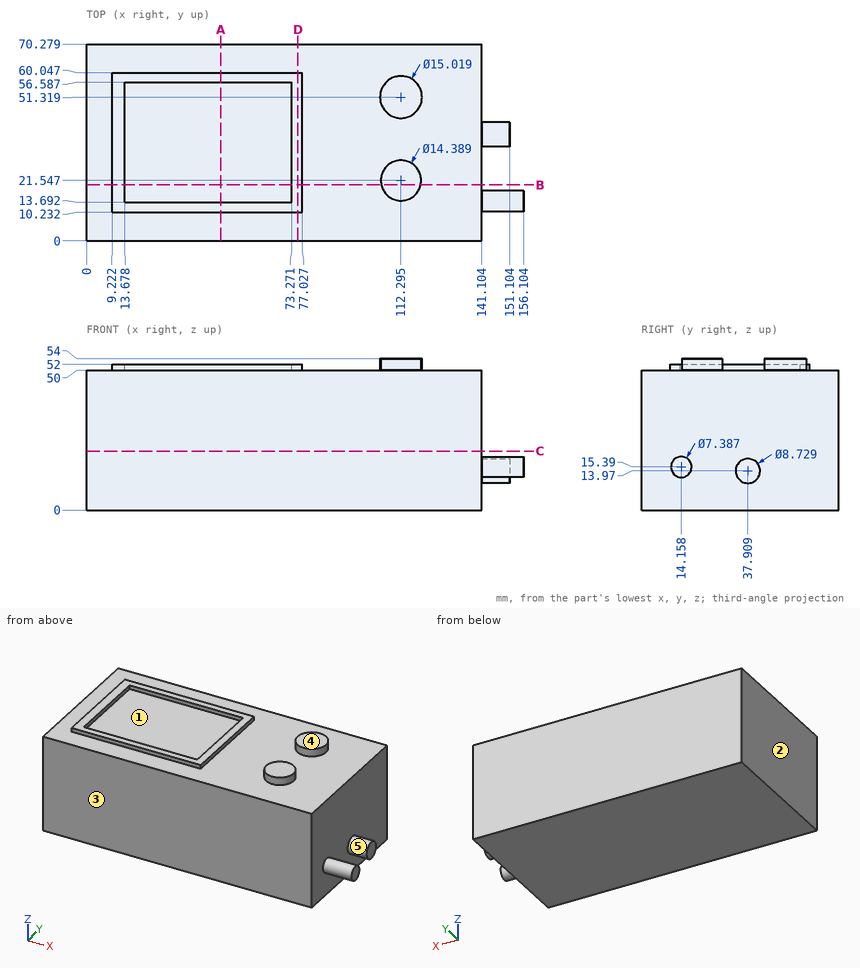
The drawing under review shows one solid part. Ordinate dimensions are in mm from its lowest x, y, z. A direction names the side the tool comes from. Give positions to 0.01 mm unless a question says otherwise; leave off trailing zeros. Write each loop counter-clockwise with the first axis right and the second up, starting at its lowest first coordinate (ties: lowest second). Pieces come first, ordered by that corner, then holes. Notation, with made-up numbers: (-11.5, -2) -> (12.5, -2) arc R37 cw to (12.5, 34) -> close; hole circle Ø9 at (57, 74). An arc over 180 degrees is marked (long way). Answer in a Markdown table with one row per item.
(1) Clearance check with flat-ended pins moving along their axes: pin 1 (1.5 mm diameter, centred on x = 94, y = 58.5, fed in from +Z); pin 2 (4.5 mm diameter, centred on y = 36.5, z = 15.5, fed in from +X) (1 decimal); pin 3 (2 mm diameter, centred on x = 44.5, z = 51.5, fed in from +Y). State where each tip first meets the part, or that it passes through.
Results:
| item | result |
|---|---|
| pin 1 | z = 50 |
| pin 2 | x = 151.1 |
| pin 3 | y = 60.05 |
(2) For the marked faces 1 and 2, list the 3-axis set-ups (+Z, -Z, +X, -X, +Y, -Y) from which the entire face can be reached by the end or side of a thin tool; tool diameter is ignored.
Results:
| item | result |
|---|---|
| face 1 | +Z |
| face 2 | +Z, -Z, -X, +Y, -Y |
(3) Consider section A-A (x = 48). State the section outline as (y, z) points.
Results:
| item | result |
|---|---|
| outline | (0, 0) -> (70.28, 0) -> (70.28, 50) -> (60.05, 50) -> (60.05, 52) -> (56.59, 52) -> (56.59, 50) -> (13.69, 50) -> (13.69, 52) -> (10.23, 52) -> (10.23, 50) -> (0, 50) -> close |
(4) Mouldability with a two-part tool opening along Y and no side actions: class the marked faces 3, 4 and 5 as +Y half, -Y half, draft (parallel to the pull), parting line (faces both ways), or undercut.
Results:
| item | result |
|---|---|
| face 3 | -Y half |
| face 4 | draft |
| face 5 | undercut |
(5) Consider section C-C (z = 21). State the section outline as (x, y) points (1 decimal).
Results:
| item | result |
|---|---|
| outline | (0, 0) -> (141.1, 0) -> (141.1, 70.3) -> (0, 70.3) -> close |
(6) Consider section B-B (y = 20). State the section outline as (x, z) points (1 decimal), then the cut area to 3 significant figures.
Results:
| item | result |
|---|---|
| outline | (0, 0) -> (141.1, 0) -> (141.1, 50) -> (119.3, 50) -> (119.3, 54) -> (105.3, 54) -> (105.3, 50) -> (77, 50) -> (77, 52) -> (73.3, 52) -> (73.3, 50) -> (13.7, 50) -> (13.7, 52) -> (9.2, 52) -> (9.2, 50) -> (0, 50) -> close |
| area | 7,130 mm2 |
(7) Consider section D-D (x = 75.5). State the section outline as (y, z) points, then the cut area to 3 significant figures.
Results:
| item | result |
|---|---|
| outline | (0, 0) -> (70.28, 0) -> (70.28, 50) -> (60.05, 50) -> (60.05, 52) -> (10.23, 52) -> (10.23, 50) -> (0, 50) -> close |
| area | 3,610 mm2 |
(8) To check wall thickness, follow probe 1 along X at (y, z) = (30, 32) (1 decimal); probe 2 along Z at (x, y) = (76.5, 48); probe 3 along Z at (x, y) = (34, 6). State the ranges of each line that lie inside material, in increasing order.
Results:
| item | result |
|---|---|
| probe 1 | 0 to 141.1 |
| probe 2 | 0 to 52 |
| probe 3 | 0 to 50 |
